Geometry check sheet. Reference: drawing and pictorial views, mm from the part's lowest x, y, z. A direction names the side the tool comes from. Round coordinates to 2 decimals unless told otherwise and drop trailing zeros. Write each loop counter-clockwise with the first axis right and the second up, starting at its lowest first coordinate (ties: lowest second). Pieces come first, ordered by that corner, then holes. Notation, with made-up numbers: M -18,22.25 L 32,22.25 A9 ccw 32,37.25 Z; hole C 39,-13 d11. An arc over 180 degrees is marked long. Answer in a Markdown table with one row per item.
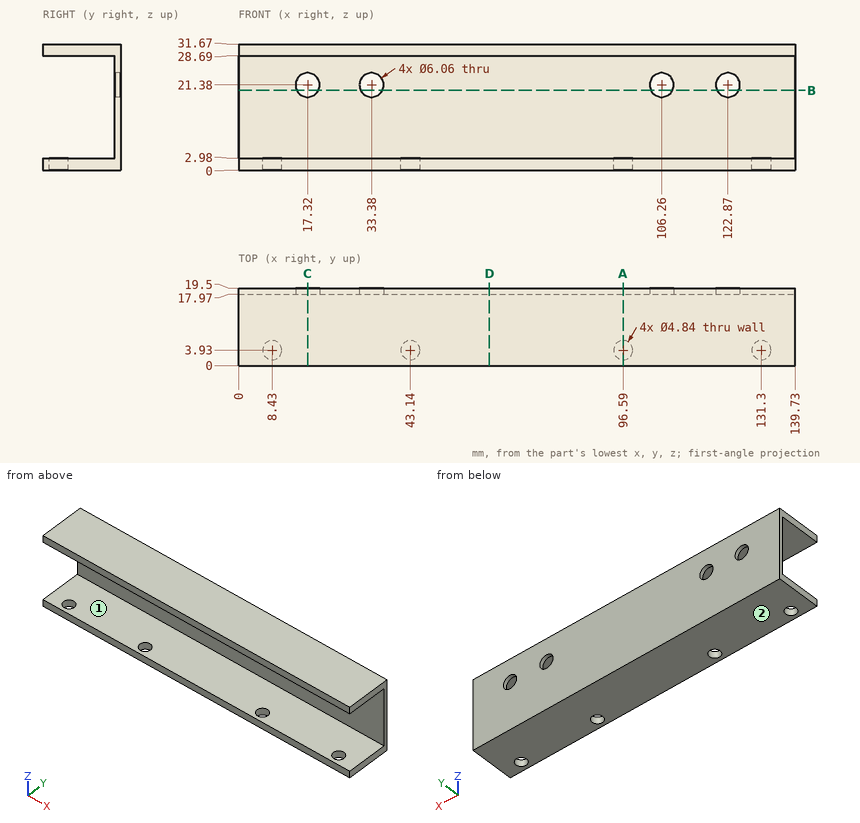
1. Section check A-A, the plane x = 96.59. Record the cut outline in (y, z), and give its area (3 significant figures).
Found:
| item | result |
|---|---|
| outline | M 0,0 L 1.51,0 L 1.51,2.98 L 0,2.98 Z; M 0,28.69 L 17.97,28.69 L 17.97,2.98 L 6.35,2.98 L 6.35,0 L 19.5,0 L 19.5,31.67 L 0,31.67 Z |
| area | 141 mm2 |
2. Go/stop test with flat-tipped pins: pin 1 (5.5 mm diameter, centred on x = 33.38, z = 21.38, fed in from -Y); pin 2 (4 mm diameter, centred on x = 43.14, y = 3.93, fed in from -Z); pin 3 (12 mm diameter, centred on x = 112.5, z = 9.5, fed in from -Y). Record where each tip stops, or that it passes through.
Found:
| item | result |
|---|---|
| pin 1 | passes through |
| pin 2 | stops at z = 28.69 |
| pin 3 | stops at y = 17.97 |
3. Section check B-B, the plane z = 20. Record the cut outline in (x, y), and give its area (3 significant figures).
Found:
| item | result |
|---|---|
| outline | M 0,17.97 L 14.62,17.97 L 14.62,19.5 L 0,19.5 Z; M 20.02,17.97 L 30.68,17.97 L 30.68,19.5 L 20.02,19.5 Z; M 36.08,17.97 L 103.56,17.97 L 103.56,19.5 L 36.08,19.5 Z; M 108.96,17.97 L 120.17,17.97 L 120.17,19.5 L 108.96,19.5 Z; M 125.57,17.97 L 139.73,17.97 L 139.73,19.5 L 125.57,19.5 Z |
| area | 181 mm2 |
4. Scan lines: L1, parallel to Z at x = 105, y = 3.25; L2, parallel to Y at x = 84, z = 9; L3, parallel to Y at x = 43.14, z = 1. Record each from-to range of solid material in increasing order.
Found:
| item | result |
|---|---|
| L1 | z = 0 to 2.98, 28.69 to 31.67 |
| L2 | y = 17.97 to 19.5 |
| L3 | y = 0 to 1.51, 6.35 to 19.5 |
5. Section check C-C, the plane x = 17.32. Record the cut outline in (y, z).
Found:
| item | result |
|---|---|
| outline | M 0,0 L 19.5,0 L 19.5,18.35 L 17.97,18.35 L 17.97,2.98 L 0,2.98 Z; M 0,28.69 L 17.97,28.69 L 17.97,24.41 L 19.5,24.41 L 19.5,31.67 L 0,31.67 Z |
6. Access from +Z, -Z, +X, -X, +Y, -Y to the whole of each face (thin tool, end or side, straight path). Record for the marked faces 1 and 2.
Found:
| item | result |
|---|---|
| face 1 | +X, -X, -Y |
| face 2 | -Z, +X, -X, +Y, -Y |
7. Section check D-D, the plane x = 63. Record the cut outline in (y, z).
Found:
| item | result |
|---|---|
| outline | M 0,0 L 19.5,0 L 19.5,31.67 L 0,31.67 L 0,28.69 L 17.97,28.69 L 17.97,2.98 L 0,2.98 Z |
